Check sheet for the modelled part. Datum: model origin and axes. Units: mm. Give positions to 0.01 mm unless a question says otherwise; leave off trailing zeros. Order: outer loops, then holes, each group sorted by start corner. A loop starts at its lowest first (then second) coordinate and runs counter-clockwise, first axis right, second up. Notation, with made-up numbers: M -0.5,-33 L 3.5,-33 A9 ccw 3.5,-18 Z; hole C 82,75.5 d1. An arc over 180 degrees is marked long. Answer in a Markdown table with one row per item. Add a question column.
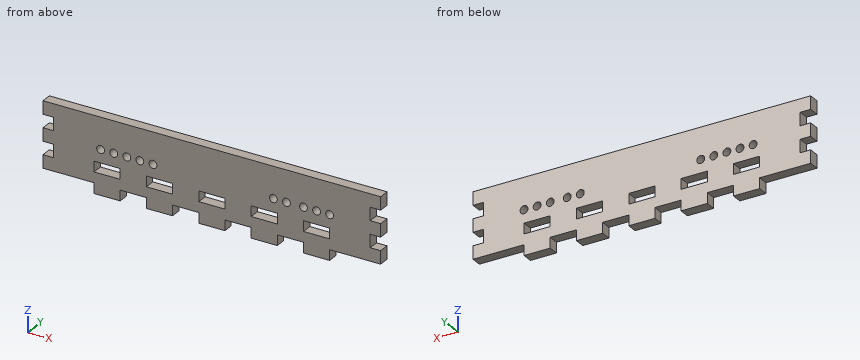
from build123d import *

# Parameters (mm, degrees)
SKETCH1_W           = 121
SKETCH1_H           = 25
BOSS_EXTRUDE1_DEPTH = 4
SKETCH2_W           = 4
SKETCH2_H           = 5
BOSS_EXTRUDE2_DEPTH = 4
LPATTERN1_COUNT     = 3
LPATTERN1_PITCH     = 10
SKETCH3_W           = 10
SKETCH3_H           = 4
BOSS_EXTRUDE3_DEPTH = 4
LPATTERN2_COUNT     = 3
LPATTERN2_PITCH     = 20
LPATTERN2_COL_COUNT = 3
LPATTERN2_COL_PITCH = 20
SKETCH4_W           = 10
SKETCH4_H           = 4
CUT_EXTRUDE1_DEPTH  = 128.538229563
SKETCH6_R           = 1.5
CUT_EXTRUDE3_DEPTH  = 128.538229563


with BuildPart() as part:
    # Sketch1 → Boss-Extrude1 (new body)
    with BuildSketch(Plane(origin=(0, 0, 0), x_dir=(1, 0, 0), z_dir=(0, 1, 0))):
        with Locations((60.5, -12.5)):
            Rectangle(SKETCH1_W, SKETCH1_H)
    extrude(amount=BOSS_EXTRUDE1_DEPTH)

    # Sketch2 → Boss-Extrude2 (add, through all)
    with BuildSketch(Plane(origin=(0, 0, 0), x_dir=(-1, 0, 0), z_dir=(0, -1, 0))):
        with Locations((2, -22.5)):
            Rectangle(SKETCH2_W, SKETCH2_H)
        with Locations((-123, -22.5)):
            Rectangle(SKETCH2_W, SKETCH2_H)
    boss_extrude2 = extrude(amount=-BOSS_EXTRUDE2_DEPTH)

    # LPattern1: Boss-Extrude2 ×3
    with Locations(*[(0, 0, -i * LPATTERN1_PITCH) for i in range(1, LPATTERN1_COUNT)]):
        add(boss_extrude2)

    # Sketch3 → Boss-Extrude3 (add, through all)
    with BuildSketch(Plane(origin=(0, 0, 0), x_dir=(-1, 0, 0), z_dir=(0, -1, 0))):
        with Locations((-60.5, 2)):
            Rectangle(SKETCH3_W, SKETCH3_H)
    boss_extrude3 = extrude(amount=-BOSS_EXTRUDE3_DEPTH)

    # LPattern2: Boss-Extrude3 ×3
    with Locations(*[(i * LPATTERN2_PITCH, 0, 0) for i in range(1, LPATTERN2_COUNT)]):
        add(boss_extrude3)

    # LPattern2 col: Boss-Extrude3 ×3
    with Locations(*[(-i * LPATTERN2_COL_PITCH, 0, 0) for i in range(1, LPATTERN2_COL_COUNT)]):
        add(boss_extrude3)

    # Sketch4 → Cut-Extrude1 (cut, through all)
    with BuildSketch(Plane.XZ):
        with Locations((20.5, 6)):
            Rectangle(SKETCH4_W, SKETCH4_H)
        with Locations((40.5, 6)):
            Rectangle(SKETCH4_W, SKETCH4_H)
        with Locations((60.5, 6)):
            Rectangle(SKETCH4_W, SKETCH4_H)
        with Locations((80.5, 6)):
            Rectangle(SKETCH4_W, SKETCH4_H)
        with Locations((100.5, 6)):
            Rectangle(SKETCH4_W, SKETCH4_H)
    extrude(amount=-CUT_EXTRUDE1_DEPTH, mode=Mode.SUBTRACT)

    # Sketch6 → Cut-Extrude3 (cut, through all)
    with BuildSketch(Plane.XZ):
        with Locations(Location((38, 13, 0), (0, 0, 270))):
            Circle(SKETCH6_R)
        with Locations(Location((33, 13, 0), (0, 0, 270))):
            Circle(SKETCH6_R)
        with Locations(Location((28, 13, 0), (0, 0, 270))):
            Circle(SKETCH6_R)
        with Locations(Location((23, 13, 0), (0, 0, 270))):
            Circle(SKETCH6_R)
        with Locations(Location((18, 13, 0), (0, 0, 270))):
            Circle(SKETCH6_R)
        with Locations(Location((84, 13, 0), (0, 0, 270))):
            Circle(SKETCH6_R)
        with Locations(Location((89, 13, 0), (0, 0, 270))):
            Circle(SKETCH6_R)
        with Locations(Location((95.5, 13, 0), (0, 0, 270))):
            Circle(SKETCH6_R)
        with Locations(Location((100.5, 13, 0), (0, 0, 270))):
            Circle(SKETCH6_R)
        with Locations(Location((105.5, 13, 0), (0, 0, 270))):
            Circle(SKETCH6_R)
    extrude(amount=-CUT_EXTRUDE3_DEPTH, mode=Mode.SUBTRACT)


solid = part.part
Q1. Cross-section at B-B (z = 13). State how many separate pieces and enclosed holes the cut face has, and give its area (3 significant figures).
Q2. Go/stop test with flat-tipped pins: pin 1 (1.2 mm diameter, centred on x = 68.5, y = 3, fed in from -Z); pin 2 (2.5 mm diameter, centred on x = 18, z = 13, fed in from -Y). Record where each tip stops, or that it passes through.
Q3. Cross-section at A-A (x = 18). Record the boundary of the cut face in (y, z), and give its area (3 significant figures).
Q4. Thickness scan on probe 1 along X at (y, z) = (2.55, -2); probe 2 along Z at (x, y) = (100.5, 1.25); probe 3 along Z at (x, y) = (89, 1.3). Record the ranges inside material, lowest first.
Values follow:
| question | item | result |
|---|---|---|
| 1 | separate pieces | 11 |
| 1 | enclosed holes | 0 |
| 1 | area | 396 mm² |
| 2 | pin 1 | z = 0 |
| 2 | pin 2 | through |
| 3 | outline | M 0,-4 L 4,-4 L 4,4 L 0,4 Z; M 0,8 L 4,8 L 4,11.5 L 0,11.5 Z; M 0,14.5 L 4,14.5 L 4,25 L 0,25 Z |
| 3 | area | 88.0 mm² |
| 4 | probe 1 | 15.5 to 25.5, 35.5 to 45.5, 55.5 to 65.5, 75.5 to 85.5, 95.5 to 105.5 |
| 4 | probe 2 | -4 to 4, 8 to 11.5, 14.5 to 25 |
| 4 | probe 3 | 0 to 11.5, 14.5 to 25 |
